from build123d import *

# Parameters (mm, degrees)
SKETCH1_W                = 1.5
SKETCH1_H                = 25
SKETCH1_W_2              = 14
SKETCH1_H_2              = 26
SKETCH1_R                = 2
BOSS_EXTRUDE1_DEPTH      = 10
SKETCH1_3_W              = 1.5
SKETCH1_3_H              = 25
BOSS_EXTRUDE2_DEPTH      = 18
SKETCH1_4_R              = 2
BOSS_EXTRUDE3_DEPTH      = 5
BOSS_EXTRUDE4_DEPTH      = 25
CUT_EXTRUDE1_DEPTH       = 4.7
CUT_EXTRUDE2_DEPTH       = 7
SKETCH8_W                = 10
SKETCH8_H                = 19
CUT_EXTRUDE3_DEPTH       = 5
MOVE_START               = -12.5
MOVE_FACE1_DEPTH         = 20.3
MOVE_START_2             = -5
MOVE_FACE1_2_OUTLINE_R   = 2
MOVE_FACE1_2_OUTLINE_R_2 = 1.85
MOVE_FACE1_2_DEPTH       = 5
MOVE_FACE1_3_OUTLINE_R   = 1.85
MOVE_FACE1_3_DEPTH       = 0.15
MOVE_FACE2_BY            = 0.1
MOVE_FACE2_2_BY          = 0.1
MOVE_FACE2_3_BY          = 0.1
MOVE_FACE2_4_BY          = 0.1
MOVE_FACE2_5_BY          = 0.1
MOVE_FACE2_6_BY          = 0.1
MOVE_FACE2_7_BY          = 0.1
MOVE_FACE2_8_BY          = 0.1
MOVE_FACE2_9_BY          = 0.1
MOVE_FACE2_10_BY         = 0.1


# Read off the part's stored shape, not the designer's step: Move Face1
with BuildPart() as part:
    # Sketch1 → Boss-Extrude1 (new body)
    # profile 1 of 5: a face of its own
    with BuildSketch(Plane.XY):
        Polygon((-7, 12.5), (-46.5, 12.5), (-46.5, -12.5), (46.5, -12.5), (46.5, 12.5), (7, 12.5), align=None)
    # profile 2 of 5: a face of its own
    with BuildSketch(Plane.XY):
        with Locations((-47.25, 0)):
            Rectangle(SKETCH1_W, SKETCH1_H)
    # profile 3 of 5: a face of its own
    with BuildSketch(Plane.XY):
        with Locations((47.25, 0)):
            Rectangle(SKETCH1_W, SKETCH1_H)
    # profile 4 of 5: a face of its own
    with BuildSketch(Plane.XY):
        with Locations((0, 25.5)):
            Rectangle(SKETCH1_W_2, SKETCH1_H_2)
        with Locations((0, 31.5)):
            Circle(SKETCH1_R, mode=Mode.SUBTRACT)
    # profile 5 of 5: a face of its own
    with BuildSketch(Plane.XY):
        with Locations((0, 31.5)):
            Circle(SKETCH1_R)
    extrude(amount=BOSS_EXTRUDE1_DEPTH)

    # Sketch1<3> → Boss-Extrude2 (add)
    with BuildSketch(Plane.XY):
        with Locations((47.25, 0)):
            Rectangle(SKETCH1_3_W, SKETCH1_3_H)
        with Locations((-47.25, 0)):
            Rectangle(SKETCH1_3_W, SKETCH1_3_H)
    extrude(amount=-BOSS_EXTRUDE2_DEPTH)

    # Sketch1<4> → Boss-Extrude3 (add)
    with BuildSketch(Plane.XY):
        with Locations((0, 31.5)):
            Circle(SKETCH1_4_R)
    extrude(amount=-BOSS_EXTRUDE3_DEPTH)

    # Sketch5 → Boss-Extrude4 (add)
    with BuildSketch(Plane(origin=(0, 12.5, 0), x_dir=(1, 0, 0), z_dir=(0, 1, 0))):
        Polygon((45.9, 17.4), (45.9, 16.6), (46.5, 16), (46.5, 18), align=None)
        Polygon((-45.9, 17.4), (-46.5, 18), (-46.5, 16), (-45.9, 16.6), align=None)
    extrude(amount=-BOSS_EXTRUDE4_DEPTH)

    # Sketch7 → Cut-Extrude1 (cut)
    with BuildSketch(Plane(origin=(0, 12.5, 0), x_dir=(1, 0, 0), z_dir=(0, 1, 0))):
        Polygon((46.5, 16), (46.5, 0), (48, 0), (48, 18), (46.5, 18), (45.9, 17.4), (45.9, 16.6), align=None)
    extrude(amount=-CUT_EXTRUDE1_DEPTH, mode=Mode.SUBTRACT)

    # Sketch7<4> → Cut-Extrude2 (cut)
    with BuildSketch(Plane(origin=(0, 12.5, 0), x_dir=(1, 0, 0), z_dir=(0, 1, 0))):
        Polygon((-48, 0), (-46.5, 0), (-46.5, 16), (-45.9, 16.6), (-45.9, 17.4), (-46.5, 18), (-48, 18), align=None)
    extrude(amount=-CUT_EXTRUDE2_DEPTH, mode=Mode.SUBTRACT)

    # Sketch8 → Cut-Extrude3 (cut)
    with BuildSketch(Plane.XY.offset(10)):
        with Locations((-27.5, 0)):
            Rectangle(SKETCH8_W, SKETCH8_H)
        with Locations((27.5, 0)):
            Rectangle(SKETCH8_W, SKETCH8_H)
    extrude(amount=-CUT_EXTRUDE3_DEPTH, mode=Mode.SUBTRACT)

    # Move Face1 outline → Move Face1 (cut)
    with BuildSketch(Plane(origin=(0, 0, 0), x_dir=(1, 0, 0), z_dir=(0, 1, 0)).offset(MOVE_START)):
        Polygon((-46.05, 16.662132034), (-46.65, 16.062132034), (-46.65, 0), (-46.5, 0), (-46.5, 16), (-45.9, 16.6), (-45.9, 17.4), (-46.5, 18), (-46.712132034, 18), (-46.05, 17.337867966), align=None)
        Polygon((46.5, 16), (46.5, 0), (46.65, 0), (46.65, 16.062132034), (46.05, 16.662132034), (46.05, 17.337867966), (46.712132034, 18), (46.5, 18), (45.9, 17.4), (45.9, 16.6), align=None)
    extrude(amount=MOVE_FACE1_DEPTH, mode=Mode.SUBTRACT)

    # Move Face1 2 outline → Move Face1 2 (cut)
    with BuildSketch(Plane.XY.offset(MOVE_START_2)):
        with Locations((0, 31.5)):
            Circle(MOVE_FACE1_2_OUTLINE_R)
        with Locations((0, 31.5)):
            Circle(MOVE_FACE1_2_OUTLINE_R_2, mode=Mode.SUBTRACT)
    extrude(amount=MOVE_FACE1_2_DEPTH, mode=Mode.SUBTRACT)

    # Move Face1 3 outline → Move Face1 3 (cut)
    with BuildSketch(Plane.XY.offset(MOVE_START_2)):
        with Locations((0, 31.5)):
            Circle(MOVE_FACE1_3_OUTLINE_R)
    extrude(amount=MOVE_FACE1_3_DEPTH, mode=Mode.SUBTRACT)

    # Move Face2: a face moved inward by 0.1
    extrude(part.faces().sort_by_distance((-22.5, 0, 7.5))[0], amount=MOVE_FACE2_BY, dir=(1, 0, 0), mode=Mode.SUBTRACT)

    # Move Face2 2: a face moved inward by 0.1
    extrude(part.faces().sort_by_distance((-32.5, 0, 7.5))[0], amount=MOVE_FACE2_2_BY, dir=(-1, 0, 0), mode=Mode.SUBTRACT)

    # Move Face2 3: a face moved inward by 0.1
    extrude(part.faces().sort_by_distance((27.5, -9.5, 7.5))[0], amount=MOVE_FACE2_3_BY, dir=(0, -1, 0), mode=Mode.SUBTRACT)

    # Move Face2 4: a face moved inward by 0.1
    extrude(part.faces().sort_by_distance((22.5, 0, 7.5))[0], amount=MOVE_FACE2_4_BY, dir=(-1, 0, 0), mode=Mode.SUBTRACT)

    # Move Face2 5: a face moved inward by 0.1
    extrude(part.faces().sort_by_distance((32.5, 0, 7.5))[0], amount=MOVE_FACE2_5_BY, dir=(1, 0, 0), mode=Mode.SUBTRACT)

    # Move Face2 6: a face moved inward by 0.1
    extrude(part.faces().sort_by_distance((27.5, 9.5, 7.5))[0], amount=MOVE_FACE2_6_BY, dir=(0, 1, 0), mode=Mode.SUBTRACT)

    # Move Face2 7: a face moved inward by 0.1
    extrude(part.faces().sort_by_distance((27.5, 0, 5))[0], amount=MOVE_FACE2_7_BY, dir=(0, 0, -1), mode=Mode.SUBTRACT)

    # Move Face2 8: a face moved inward by 0.1
    extrude(part.faces().sort_by_distance((-27.5, -9.5, 7.5))[0], amount=MOVE_FACE2_8_BY, dir=(0, -1, 0), mode=Mode.SUBTRACT)

    # Move Face2 9: a face moved inward by 0.1
    extrude(part.faces().sort_by_distance((-27.5, 9.5, 7.5))[0], amount=MOVE_FACE2_9_BY, dir=(0, 1, 0), mode=Mode.SUBTRACT)

    # Move Face2 10: a face moved inward by 0.1
    extrude(part.faces().sort_by_distance((-27.5, 0, 5))[0], amount=MOVE_FACE2_10_BY, dir=(0, 0, -1), mode=Mode.SUBTRACT)


solid = part.part
Source: CAD feature listing. Evaluate the final solid. Frame: model axes, mm. A direction names the side the tool comes from. Coordinates: 2 decimals unless noted, no trailing zeros. Loops run counter-clockwise (first coordinate to the right, second up) from the corner with the lowest first, then second, coordinate; pieces in that order, holes last. Notation, with made-up numbers: (89.25, 75.25) - (122.25, 75.25) arc R16 ccw to (122.25, 98.25) - close; hole circle Ø10 at (85, 3). An arc over 180 degrees is marked (long way). One line per item, written item: value. Start each with the question number.
1. Ray query, L1, parallel to X at y = 2.5, z = -4.75; L2, parallel to Z at x = 22, y = 2.5; L3, parallel to X at y = 7, z = -5. Return the intervals inside material, ascending.
2. Mould query, pull axis Y, two halves, no side actions, for faces 4 (the flat face through (0, 38.5, 5)), 5 (the flat face through (32.6, 0, 7)), 6 (the flat face through (-1, 2, 10)). Classes: pulls with the +Y half, pulls with the -Y half, needs draft (parallel to the pull), parting line crosses it, or undercut.
3. Contact query for flat-ended pins moving along their axis: P1, Ø1, axis at x = -47, z = -12, coming from the +Y side; P2, Ø3, axis at x = 0.5, y = 32, coming from the -Z side; P3, Ø2.5, axis at x = 28.5, z = 8.5, coming from the +Y side. Output: stop coordinate, or through.
4. Set-up query: faces 1 (the flat face through (-47, 5.5, -9)), 2 (the flat face through (-7, 25, 5)), 3 (the flat face through (-32.6, 0, 7)). Return all of +Z, -Z, +X, -X, +Y, -Y with unobstructed straight access to the full face (end or side cutting, diameter ignored); none if empty.
5. Section B-B (z = -2.75). Return the cut outline in (x, y), and give its area (3 significant figures).
6. Section C-C (x = 0). Return the cut outline in (y, z).
7. Section A-A (z = -14.25). Return the cut outline in (x, y).
8. Section D-D (y = 31.5). Return the cut outline in (x, z).
Verdict:
1. L1: x = -48 to -46.65, 46.65 to 48
1. L2: z = 0 to 10
1. L3: x = 46.65 to 48
2. face 4: pulls with the +Y half
2. face 5: undercut
2. face 6: needs draft
3. P1: stops at y = 5.5
3. P2: stops at z = -4.85
3. P3: stops at y = 12.5
4. face 1: -Z, -X, +Y
4. face 2: +Z, -Z, -X, +Y
4. face 3: +Z
5. outline: (-48, -12.5) - (-46.65, -12.5) - (-46.65, 5.5) - (-48, 5.5) - close; circle Ø3.7 at (0, 31.5); (46.65, -12.5) - (48, -12.5) - (48, 7.8) - (46.65, 7.8) - close
5. area: 62.5 mm2
6. outline: (-12.5, 0) - (29.65, 0) - (29.65, -4.85) - (33.35, -4.85) - (33.35, 0) - (38.5, 0) - (38.5, 10) - (-12.5, 10) - close
7. outline: (-48, -12.5) - (-46.65, -12.5) - (-46.65, 5.5) - (-48, 5.5) - close; (46.65, -12.5) - (48, -12.5) - (48, 7.8) - (46.65, 7.8) - close
8. outline: (-7, 0) - (-1.85, 0) - (-1.85, -4.85) - (1.85, -4.85) - (1.85, 0) - (7, 0) - (7, 10) - (-7, 10) - close
